```python
from build123d import *

# Parameters (mm, degrees)
SKETCH1_R           = 55.5
SKETCH1_R_2         = 4
BOSS_EXTRUDE4_DEPTH = 2
SKETCH6_W           = 69
SKETCH6_H           = 84
SKETCH6_W_2         = 65
SKETCH6_H_2         = 80
BOSS_EXTRUDE5_DEPTH = 15
SKETCH7_R           = 10
CUT_EXTRUDE2_DEPTH  = 30


with BuildPart() as part:
    # Sketch1 → Boss-Extrude4 (new body)
    with BuildSketch(Plane(origin=(0, 0, 0), x_dir=(1, 0, 0), z_dir=(0, 1, 0))):
        with Locations(Location((0, 0, 0), (0, 0, 270))):
            Circle(SKETCH1_R)
        with Locations(Location((0, 49.5, 0), (0, 0, 270))):
            Circle(SKETCH1_R_2, mode=Mode.SUBTRACT)
        with Locations(Location((49.5, 0, 0), (0, 0, 270))):
            Circle(SKETCH1_R_2, mode=Mode.SUBTRACT)
        with Locations(Location((-49.5, 0, 0), (0, 0, 270))):
            Circle(SKETCH1_R_2, mode=Mode.SUBTRACT)
        with Locations(Location((0, -49.5, 0), (0, 0, 270))):
            Circle(SKETCH1_R_2, mode=Mode.SUBTRACT)
    extrude(amount=BOSS_EXTRUDE4_DEPTH)

    # Sketch6 → Boss-Extrude5 (add)
    with BuildSketch(Plane(origin=(0, 2, 0), x_dir=(1, 0, 0), z_dir=(0, 1, 0))):
        Rectangle(SKETCH6_W, SKETCH6_H)
        Rectangle(SKETCH6_W_2, SKETCH6_H_2, mode=Mode.SUBTRACT)
    extrude(amount=BOSS_EXTRUDE5_DEPTH)

    # Sketch7 → Cut-Extrude2 (cut)
    with BuildSketch(Plane(origin=(0, 2, 0), x_dir=(1, 0, 0), z_dir=(0, 1, 0))):
        with Locations(Location((0, 0, 0), (0, 0, 270))):
            Circle(SKETCH7_R)
    extrude(amount=-CUT_EXTRUDE2_DEPTH, mode=Mode.SUBTRACT)


solid = part.part
```
Geometry: final body of the model. Coordinates: model frame, mm. A direction names the side the tool comes from. Give positions to 0.01 mm unless a question says otherwise; leave off trailing zeros. Write each loop counter-clockwise with the first axis right and the second up, starting at its lowest first coordinate (ties: lowest second). Pieces come first, ordered by that corner, then holes.
1. Section query A-A, the plane z = 0. Return loops of the section in (x, y), then the cut area to 3 significant figures.
2. Section query C-C, the plane y = 4.5. Return loops of the section in (x, z).
3. Pin query (flat end, axial travel): P1, Ø12, axis at x = 22.5, z = -27, coming from the -Y side; P2, Ø5, axis at y = 7, z = -26.5, coming from the +X side; P3, Ø4.5, axis at x = 8, y = 8, coming from the -Z side; P4, Ø1.5, axis at x = -12.5, y = 4.5, coming from the +Z side. Return the tip coordinate at first contact, or that it passes through.
4. Reachability of faces 1 (the cylindrical face through (-2.4, 1, -52.7)), 2 (the flat face through (-12, 0, -1)), 3 (the flat face through (34.5, 9, 1)), 4 (the flat face through (8, 2, 8)), 5 (the flat face through (0, 9, -42)) from +Z, -Z, +X, -X, +Y, -Y: full face, straight path, thin tool, end or side. Return the list, or none.
5. Draft query along Z for faces 6 (the flat face through (-32.5, 9, 1)), 7 (the flat face through (-34.5, 9, 1)), 8 (the flat face through (0, 9, 42)), 9 (the flat face through (0, 9, 40)). Return one class per face: released by +Z, released by -Z, zero draft, split by the parting line, or undercut.
6. Section query B-B, the plane x = -49.5. Return loops of the section in (y, z), then the cut area to 3 significant figures.
7. Line query: probe 1 along X at (y, z) = (1.35, 0); probe 2 along Z at (x, y) = (-19.5, 15); probe 3 along X at (y, z) = (15.5, -9). Output: solid intervals per line, ascending.
8. Section query D-D, the plane z = -49.5. Return loops of the section in (x, y).
Computed:
1. outline: (-55.5, 0) - (-53.5, 0) - (-53.5, 2) - (-55.5, 2) - close; (-45.5, 0) - (-10, 0) - (-10, 2) - (-32.5, 2) - (-32.5, 17) - (-34.5, 17) - (-34.5, 2) - (-45.5, 2) - close; (10, 0) - (45.5, 0) - (45.5, 2) - (34.5, 2) - (34.5, 17) - (32.5, 17) - (32.5, 2) - (10, 2) - close; (53.5, 0) - (55.5, 0) - (55.5, 2) - (53.5, 2) - close
1. area: 210 mm2
2. outline: (-34.5, -42) - (34.5, -42) - (34.5, 42) - (-34.5, 42) - close; hole (-32.5, -40) - (32.5, -40) - (32.5, 40) - (-32.5, 40) - close
3. P1: stops at y = 0
3. P2: stops at x = 34.5
3. P3: stops at z = -42
3. P4: stops at z = 42
4. face 1: +Y, -Y
4. face 2: +Z, -Z, +X, -X, -Y
4. face 3: +Z, -Z, +X, +Y
4. face 4: +Y
4. face 5: -Z, +X, -X, +Y
5. face 6: undercut
5. face 7: zero draft
5. face 8: released by +Z
5. face 9: undercut
6. outline: (0, -25.1) - (2, -25.1) - (2, -4) - (0, -4) - close; (0, 4) - (2, 4) - (2, 25.1) - (0, 25.1) - close
6. area: 84.4 mm2
7. probe 1: x = -55.5 to -53.5, -45.5 to -10, 10 to 45.5, 53.5 to 55.5
7. probe 2: z = -42 to -40, 40 to 42
7. probe 3: x = -34.5 to -32.5, 32.5 to 34.5
8. outline: (-25.1, 0) - (-4, 0) - (-4, 2) - (-25.1, 2) - close; (4, 0) - (25.1, 0) - (25.1, 2) - (4, 2) - close
